```python
from build123d import *

# Parameters (mm, degrees)
SKETCH1_W           = 15
SKETCH1_H           = 22.5
BOSS_EXTRUDE1_DEPTH = 15
SKETCH2_R           = 2
CUT_EXTRUDE1_DEPTH  = 31.923292192
SKETCH3_R           = 2
CUT_EXTRUDE2_DEPTH  = 31.923292192
SKETCH4_R           = 3.5
CUT_EXTRUDE3_DEPTH  = 4
SKETCH5_R           = 3.5
CUT_EXTRUDE4_DEPTH  = 4


with BuildPart() as part:
    # Sketch1 → Boss-Extrude1 (new body)
    with BuildSketch(Plane(origin=(0, 0, 0), x_dir=(1, 0, 0), z_dir=(0, 1, 0))):
        with Locations((7.5, 11.25)):
            Rectangle(SKETCH1_W, SKETCH1_H)
    extrude(amount=BOSS_EXTRUDE1_DEPTH)

    # Sketch2 → Cut-Extrude1 (cut, through all)
    with BuildSketch(Plane(origin=(0, 15, 0), x_dir=(1, 0, 0), z_dir=(0, 1, 0))):
        with Locations(Location((7.5, 6.25, 0), (0, 0, 270))):
            Circle(SKETCH2_R)
    extrude(amount=-CUT_EXTRUDE1_DEPTH, mode=Mode.SUBTRACT)

    # Sketch3 → Cut-Extrude2 (cut, through all)
    with BuildSketch(Plane.ZY):
        with Locations((-16.25, 7.5)):
            Circle(SKETCH3_R)
    extrude(amount=-CUT_EXTRUDE2_DEPTH, mode=Mode.SUBTRACT)

    # Sketch4 → Cut-Extrude3 (cut)
    with BuildSketch(Plane(origin=(0, 15, 0), x_dir=(1, 0, 0), z_dir=(0, 1, 0))):
        with Locations(Location((7.5, 6.25, 0), (0, 0, 270))):
            Circle(SKETCH4_R)
    extrude(amount=-CUT_EXTRUDE3_DEPTH, mode=Mode.SUBTRACT)

    # Sketch5 → Cut-Extrude4 (cut)
    with BuildSketch(Plane(origin=(15, 0, 0), x_dir=(0, 0, -1), z_dir=(1, 0, 0))):
        with Locations((16.25, 7.5)):
            Circle(SKETCH5_R)
    extrude(amount=-CUT_EXTRUDE4_DEPTH, mode=Mode.SUBTRACT)


solid = part.part
```
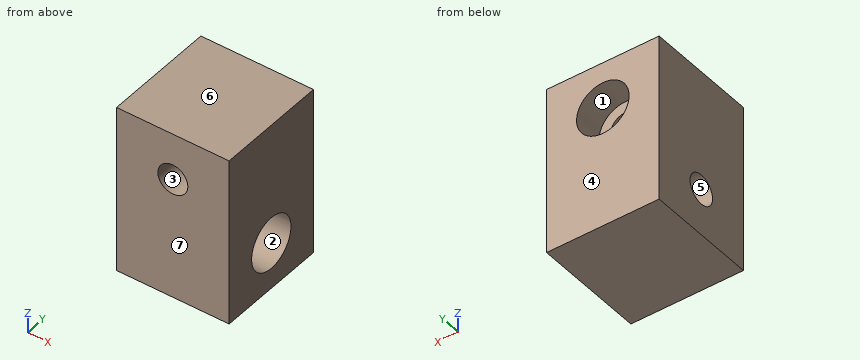
For this review, take the finished solid that the model builds, in its own axes (mm). Face numbers are marked on the shaded views. A direction names the side the tool comes from. Coordinates: 2 decimals unless noted, no trailing zeros. Write each loop counter-clockwise with the first axis right and the second up, starting at its lowest first coordinate (ties: lowest second). Pieces come first, ordered by that corner, then holes.
(1) Add section D-D on x = 11.5. Give the boundary of the cut face in (y, z), then the cut area to 3 significant figures.
(2) Add section B-B on x = 6. Give the boundary of the cut face in (y, z), then the cut area to 3 significant figures.
(3) Add section C-C on z = -16.25. Give the boundary of the cut face in (x, y).
(4) Wall thickness on probe 1 along Y at (x, z) = (3, -16.25); probe 2 along Y at (x, z) = (12.05, -16.25): over which ranges is each line inside the solid? List them lowest first.
(5) The part is to be moulded in two halves that separate along Y. For the marked faces 4, 5, 6 and 7, say which applies: +Y half, -Y half, draft (parallel to the pull), parting line (faces both ways), or undercut.
(6) For pin 1 Ø3 at (x, z) = (9.5, -9.5) entering from -Y; pin 2 Ø2 at (y, z) = (9, -16) entering from +X, all flat-tipped, find the tip position at first contact; note any pin that passes through.
(7) Tool access review of the marked faces 1, 2 and 3: name each direction out of +Z, -Z, +X, -X, +Y, -Y from which nothing blocks a thin tool from reaching the whole face with its end or side.
(8) Add section A-A on y = 7.5. Give the boundary of the cut face in (x, z).
Answer sheet:
1. outline: (0, -22.5) - (15, -22.5) - (15, 0) - (0, 0) - close; hole circle Ø7 at (7.5, -16.25)
1. area: 299 mm2
2. outline: (0, -22.5) - (15, -22.5) - (15, -9.41) - (11, -9.41) - (11, -7.57) - (0, -7.57) - close; (0, -4.93) - (11, -4.93) - (11, -3.09) - (15, -3.09) - (15, 0) - (0, 0) - close; hole circle Ø4 at (7.5, -16.25)
2. area: 271 mm2
3. outline: (0, 0) - (15, 0) - (15, 4) - (11, 4) - (11, 5.5) - (0, 5.5) - close; (0, 9.5) - (11, 9.5) - (11, 11) - (15, 11) - (15, 15) - (0, 15) - close
4. probe 1: y = 0 to 5.5, 9.5 to 15
4. probe 2: y = 0 to 4, 11 to 15
5. face 4: +Y half
5. face 5: undercut
5. face 6: draft
5. face 7: -Y half
6. pin 1: stops at y = 0
6. pin 2: stops at x = 11
7. face 1: +Y
7. face 2: +X
7. face 3: +Y, -Y
8. outline: (0, -22.5) - (15, -22.5) - (15, -19.75) - (11, -19.75) - (11, -18.25) - (0, -18.25) - close; (0, -14.25) - (11, -14.25) - (11, -12.75) - (15, -12.75) - (15, 0) - (0, 0) - close; hole circle Ø4 at (7.5, -6.25)
